from build123d import *

# Parameters (mm, degrees)
F0_W            = 210
F0_H            = 225
F1_DEPTH        = 25
F3_DEPTH        = 95
F4_R            = 37.5
F5_DEPTH        = 10
F5_DEPTH_BACK   = 127
F7_DEPTH        = 10
F7_DEPTH_BACK   = 127
F8_W            = 60
F8_H            = 60
F9_DEPTH        = 10
F10_R           = 10
F12_DEPTH       = 20
F14_D           = 15
F14_CBORE_D     = 30
F14_CBORE_DEPTH = 10
F15_R           = 10
F16_R           = 19.5
F17_DEPTH       = 235.001
F18_R           = 19.5
F19_DEPTH       = 220.001
F20_R           = 5


with BuildPart() as f1:
    # F0 (on Top) → F1 (new body)
    with BuildSketch(Plane.XY):
        Rectangle(F0_W, F0_H)
    extrude(amount=F1_DEPTH)

    # F2 (on face) → F3 (join)
    with BuildSketch(Plane.XY.offset(25)):
        with BuildLine():
            Line((-71, -32.5), (-71, -112.5))
            Line((-71, -112.5), (-56, -112.5))
            Line((-56, -112.5), (-56, -46.4818166789))
            ThreePointArc((-56, -46.4818166789), (7.4888527117, -14.9888527117), (38.9818166789, 48.5))
            Line((38.9818166789, 48.5), (105, 48.5))
            Line((105, 48.5), (105, 63.5))
            Line((105, 63.5), (25, 63.5))
            ThreePointArc((25, 63.5), (-3.1177490061, -4.3822509939), (-71, -32.5))
        make_face()
    extrude(amount=F3_DEPTH)

    # F4 (on face) → F5 (join, two sides)
    with BuildSketch(Plane.XZ.offset(112.5)) as f5_sk:
        with Locations((-63.5, 120)):
            Circle(F4_R)
    extrude(amount=F5_DEPTH)
    extrude(f5_sk.sketch, amount=-F5_DEPTH_BACK)

    # F6 (on face) → F7 (join, two sides)
    with BuildSketch(Plane.YZ.offset(105)) as f7_sk:
        with BuildLine():
            Line((48.5, 120), (48.5, 80.7094158862))
            ThreePointArc((48.5, 80.7094158862), (56, 80), (63.5, 80.7094158862))
            Line((63.5, 80.7094158862), (63.5, 120))
            Line((63.5, 120), (48.5, 120))
        make_face()
        with BuildLine():
            ThreePointArc((63.5, 80.7094158862), (86.8220700148, 94.504902432), (96, 120))
            ThreePointArc((96, 120), (30.504902432, 150.8220700148), (48.5, 80.7094158862))
            Line((48.5, 80.7094158862), (48.5, 120))
            Line((48.5, 120), (63.5, 120))
            Line((63.5, 120), (63.5, 80.7094158862))
        make_face()
    extrude(amount=F7_DEPTH)
    extrude(f7_sk.sketch, amount=-F7_DEPTH_BACK)

    # F8 (on face) → F9 (join)
    with BuildSketch(Plane.XY.offset(25)):
        with Locations((75, -82.5)):
            Rectangle(F8_W, F8_H)
    extrude(amount=F9_DEPTH)

    # F10
    f10_edges = [f1.edges().sort_by_distance(p)[0] for p in [
        (45, -52.5, 30),
    ]]
    fillet(f10_edges, radius=F10_R)

    # F11 (on face) → F12 (cut)
    with BuildSketch(Plane.XY.offset(25)):
        with BuildLine():
            ThreePointArc((46.5755076536, 39.5), (13.8528137424, -21.3528137424), (-47, -54.0755076536))
            Line((-47, -54.0755076536), (-47, -103.5))
            Line((-47, -103.5), (36, -103.5))
            Line((36, -103.5), (36, -62.5))
            ThreePointArc((36, -62.5), (41.5649711575, -49.0649711575), (55, -43.5))
            Line((55, -43.5), (96, -43.5))
            Line((96, -43.5), (96, 39.5))
            Line((96, 39.5), (46.5755076536, 39.5))
        make_face()
    extrude(amount=-F12_DEPTH, mode=Mode.SUBTRACT)

    # F14 (through all)
    with Locations(Plane.XY.offset(35)):
        with Locations((75, -82.5)):
            CounterBoreHole(F14_D / 2, F14_CBORE_D / 2, F14_CBORE_DEPTH)

    # F15
    f15_edges = [f1.edges().sort_by_distance(p)[0] for p in [
        (-47, -103.5, 15),
        (96, 39.5, 15),
        (-47, -54.075508, 15),
        (46.575508, 39.5, 15),
        (96, -43.5, 15),
        (36, -103.5, 15),
    ]]
    fillet(f15_edges, radius=F15_R)

    # F16 (on face) → F17 (cut, through all)
    with BuildSketch(Plane.XZ.offset(122.5)):
        with Locations((-63.5, 120)):
            Circle(F16_R)
    extrude(amount=-F17_DEPTH, mode=Mode.SUBTRACT)

    # F18 (on face) → F19 (cut, through all)
    with BuildSketch(Plane.YZ.offset(115)):
        with Locations((56, 120)):
            Circle(F18_R)
    extrude(amount=-F19_DEPTH, mode=Mode.SUBTRACT)

    # F20
    f20_edges = [f1.edges().sort_by_distance(p)[0] for p in [
        (-105, -112.5, 12.5),
        (105, -112.5, 17.5),
        (105, 112.5, 12.5),
        (-105, 112.5, 12.5),
        (-83, 14.5, 120),
        (-22, 36.5, 120),
        (115, 36.5, 120),
        (-83, -122.5, 120),
    ]]
    fillet(f20_edges, radius=F20_R)


solid = f1.part
Geometry: final body of the model. Coordinates: model frame, mm. A direction names the side the tool comes from. Coordinates: 2 decimals unless noted, no trailing zeros. Loops run counter-clockwise (first coordinate to the right, second up) from the corner with the lowest first, then second, coordinate; pieces in that order, holes last. Notation, with made-up numbers: M -23,83.5 L 6,83.5 A20 cw 6,122.5 Z; hole C 40.25,-15 d7. An arc over 180 degrees is marked long. One line per item, written item: value. Start each with the question number.
1) Cut plane C-C (z = 71). Return loops of the section in (x, y), then the cut area to 3 significant figures.
2) Material intervals for L1, parallel to X at y = -82, z = 14; L2, parallel to Y at x = 75, z = 28; L3, parallel to Z at x = -63, y = -20, sorted ascending. Write a range as from..to.
3) Pin query (flat end, axial travel): P1, Ø8, axis at y = 79, z = 114.5, coming from the +X side; P2, Ø6, axis at y = -64.5, z = 122, coming from the -X side; P3, Ø6, axis at x = 72.5, z = 11, coming from the -Y side; P4, Ø8, axis at x = 90.5, z = 75, coming from the -Y side. Return the tip coordinate at first contact, or that it passes through.
4) Draft query along Z for faces 1 (the cylindrical face through (48.33, 37.39, 14.86)), 2 (the flat face through (80, -52.5, 30)). Return one class per face: released by +Z, released by -Z, zero draft, split by the parting line, or undercut.
5) Reachability of faces 3 (the cylindrical face through (32.99, -100.65, 14.86)), 4 (the cylindrical face through (-44.15, -100.49, 14.86)), 5 (the flat face through (-71, -72, 54)), 6 (the flat face through (-25, 27, 25)), 7 (the flat face through (45, -88, 30)) from +Z, -Z, +X, -X, +Y, -Y: full face, straight path, thin tool, end or side. Return the list, or none.
6) Cut plane A-A (y = -82.5). Return loops of the section in (x, z).
7) Cut plane B-B (x = 75). Return loops of the section in (y, z), then the cut area to 3 significant figures.
8) Cut plane D-D (x = -63.5). Return loops of the section in (y, z), then the cut area to 3 significant figures.
Evaluation:
1. outline: M -71,-112.5 L -56,-112.5 L -56,-46.48 A111 ccw 38.98,48.5 L 105,48.5 L 105,63.5 L 25,63.5 A96 cw -71,-32.5 Z
1. area: 4,400 mm^2
2. L1: -105..-47, 36..67.52, 82.48..105
2. L2: -112.5..-97.5, -67.5..-52.5, 48.5..63.5
2. L3: 0..25, 82.5..100.51, 139.49..157.5
3. P1: x = 115
3. P2: x = -101
3. P3: y = -112.5
3. P4: y = 48.5
4. face 1: undercut
4. face 2: zero draft
5. face 3: +Z
5. face 4: none
5. face 5: -X, +Y, -Y
5. face 6: -X, +Y
5. face 7: +Z, -Y
6. outline: M -105,0 L 67.5,0 L 67.5,25 L 60,25 L 60,35 L 45,35 L 45,25 L 36,25 L 36,5 L -47,5 L -47,25 L -56,25 L -56,83.26 A37.5 ccw long -71,83.26 L -71,25 L -105,25 Z; M 82.5,0 L 105,0 L 105,35 L 90,35 L 90,25 L 82.5,25 Z; hole C -63.5,120 d39
7. outline: M -112.5,0 L -90,0 L -90,25 L -97.5,25 L -97.5,35 L -112.5,35 Z; M -75,0 L 112.5,0 L 112.5,25 L 63.5,25 L 63.5,80.71 A40 ccw long 48.5,80.71 L 48.5,25 L 39.5,25 L 39.5,5 L -43.5,5 L -43.5,25 L -52.5,25 L -52.5,35 L -67.5,35 L -67.5,25 L -75,25 Z; hole C 56,120 d39
7. area: 8,550 mm^2
8. outline: M -122.5,82.5 L -112.5,82.5 L -112.5,0 L 112.5,0 L 112.5,25 L -32.21,25 L -32.21,82.5 L 14.5,82.5 L 14.5,95.5 A5 ccw 9.5,100.5 L -117.5,100.5 A5 ccw -122.5,95.5 Z; M -122.5,144.5 A5 ccw -117.5,139.5 L 9.5,139.5 A5 ccw 14.5,144.5 L 14.5,157.5 L -122.5,157.5 Z
8. area: 15,200 mm^2
